Read the model definition and answer for the solid it produces. Units are mm, in the model's axes. Round coordinates to 2 decimals unless told otherwise and drop trailing zeros. Order: outer loops, then holes, each group sorted by start corner. A loop starts at its lowest first (then second) coordinate and runs counter-clockwise, first axis right, second up. Notation, with made-up numbers: (-21, 9.5) - (25, 9.5) arc R35 ccw to (25, 41.5) - close; hole circle Ø1 at (-22.5, -21.75). An arc over 180 degrees is marked (long way). Put each result on its own line as item: value. Start each with the question number.
Q1. Section D-D on x = 108.5 is taken. Give the vertices of the cut face in (y, z), then the cut area to 3 significant figures.
Q2. Find the intervals of material crossed by line 1 along X through (y, z) = (-0.6, 109); line 2 along Z through (x, y) = (-35.5, -2.75); line 3 along Z through (x, y) = (36.5, -0.65), in increasing order. Write a range as from..to.
Q3. Section A-A on x = 0 is taken. Give the vertices of the cut face in (y, z), then the cut area to 3 significant figures.
Q4. Section B-B on z = 0 is taken. Give the vertices of the cut face in (x, y).
Q5. Each of these flat-tipped pins is pushed along its axis until it touches: pin 1 Ø22 at (x, z) = (44.01, 106.25) entering from -Y; pin 2 Ø1 at (y, z) = (-1.5, -89) entering from +X; pin 3 Ø1 at (x, y) = (10, -2.5) entering from +Z. Where does it stop, or does it pass through?
Q6. Section C-C on y = -1.3 is taken. State how many separate pieces and enclosed holes the cut face has, then the cut area to 3 significant figures.
from build123d import *

# Parameters (mm, degrees)
F0_R     = 132.5
F0_R_2   = 9.5
F0_R_3   = 82.6
F1_DEPTH = 3


with BuildPart() as f1:
    # F0 (on Front) → F1 (new body)
    with BuildSketch(Plane.XZ):
        Circle(F0_R)
        with Locations((-44.008595, -106.246146)):
            Circle(F0_R_2, mode=Mode.SUBTRACT)
        with Locations((-106.246146, -44.008595)):
            Circle(F0_R_2, mode=Mode.SUBTRACT)
        with Locations((44.008595, -106.246146)):
            Circle(F0_R_2, mode=Mode.SUBTRACT)
        with Locations((106.246146, -44.008595)):
            Circle(F0_R_2, mode=Mode.SUBTRACT)
        with Locations((-106.246146, 44.008595)):
            Circle(F0_R_2, mode=Mode.SUBTRACT)
        with Locations((-44.008595, 106.246146)):
            Circle(F0_R_2, mode=Mode.SUBTRACT)
        Circle(F0_R_3, mode=Mode.SUBTRACT)
        with Locations((106.246146, 44.008595)):
            Circle(F0_R_2, mode=Mode.SUBTRACT)
        with Locations((44.008595, 106.246146)):
            Circle(F0_R_2, mode=Mode.SUBTRACT)
    extrude(amount=F1_DEPTH)


solid = f1.part
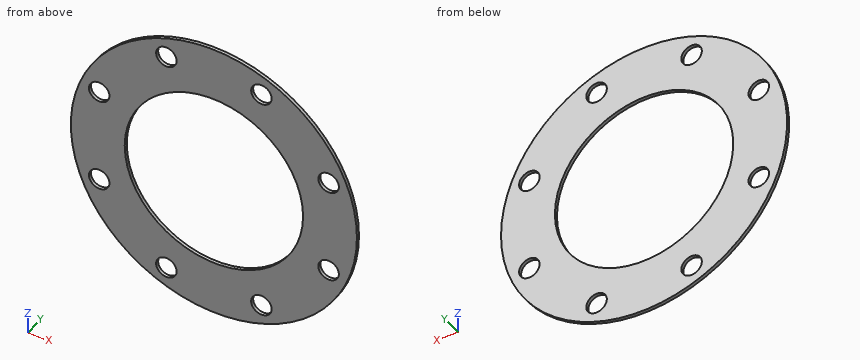
Findings:
1. outline: (-3, -76.05) - (0, -76.05) - (0, -53.24) - (-3, -53.24) - close; (-3, -34.78) - (0, -34.78) - (0, 34.78) - (-3, 34.78) - close; (-3, 53.24) - (0, 53.24) - (0, 76.05) - (-3, 76.05) - close
1. area: 346 mm2
2. line 1: -75.33..-53.1, -34.92..34.92, 53.1..75.33
2. line 2: -127.66..-110.47, -102.02..-74.58, 74.58..102.02, 110.47..127.66
2. line 3: -127.37..-112.07, -100.43..-74.1, 74.1..100.43, 112.07..127.37
3. outline: (-3, -132.5) - (0, -132.5) - (0, -82.6) - (-3, -82.6) - close; (-3, 82.6) - (0, 82.6) - (0, 132.5) - (-3, 132.5) - close
3. area: 299 mm2
4. outline: (-132.5, -3) - (-82.6, -3) - (-82.6, 0) - (-132.5, 0) - close; (82.6, -3) - (132.5, -3) - (132.5, 0) - (82.6, 0) - close
5. pin 1: y = -3
5. pin 2: x = 98.61
5. pin 3: z = 132.16
6. separate pieces: 1
6. enclosed holes: 9
6. area: 31,500 mm2
